```python
from build123d import *

# Parameters (mm, degrees)
SKETCH2_W           = 41
SKETCH2_H           = 35
BOSS_EXTRUDE1_DEPTH = 23.5
SKETCH3_W           = 30
SKETCH3_H           = 26
BOSS_EXTRUDE2_DEPTH = 5
SKETCH4_R           = 0.4
BOSS_EXTRUDE3_DEPTH = 2.5
CHAMFER1_SIZE       = 0.2


with BuildPart() as part:
    # Sketch2 → Boss-Extrude1 (new body)
    with BuildSketch(Plane(origin=(0, 0, 0), x_dir=(1, 0, 0), z_dir=(0, 1, 0))):
        Rectangle(SKETCH2_W, SKETCH2_H)
    extrude(amount=BOSS_EXTRUDE1_DEPTH)

    # Sketch3 → Boss-Extrude2 (add)
    with BuildSketch(Plane(origin=(0, 23.5, 0), x_dir=(1, 0, 0), z_dir=(0, 1, 0))):
        Rectangle(SKETCH3_W, SKETCH3_H)
    extrude(amount=BOSS_EXTRUDE2_DEPTH)

    # Sketch4 → Boss-Extrude3 (add)
    with BuildSketch(Plane.XZ):
        with Locations(Location((-10, 12.5, 0), (0, 0, 90))):
            Circle(SKETCH4_R)
        with Locations(Location((10, 12.5, 0), (0, 0, 90))):
            Circle(SKETCH4_R)
        with Locations(Location((-5, -12.5, 0), (0, 0, 90))):
            Circle(SKETCH4_R)
        with Locations(Location((5, -12.5, 0), (0, 0, 90))):
            Circle(SKETCH4_R)
    extrude(amount=BOSS_EXTRUDE3_DEPTH)

    # Chamfer1
    chamfer1_edges = [part.edges().sort_by_distance(p)[0] for p in [
        (20.5, 23.5, 0),
        (0, 23.5, -17.5),
        (15, 26, 13),
        (-15, 26, -13),
        (-15, 26, 13),
        (15, 28.5, 0),
        (0, 28.5, -13),
        (-15, 28.5, 0),
        (0, 28.5, 13),
        (-20.5, 23.5, 0),
        (0, 23.5, 17.5),
        (-20.5, 11.75, -17.5),
        (20.5, 11.75, -17.5),
        (20.5, 11.75, 17.5),
        (-20.5, 11.75, 17.5),
    ]]
    chamfer(chamfer1_edges, length=CHAMFER1_SIZE)


solid = part.part
```
For this review, take the finished solid that the model builds, in its own axes (mm). A direction names the side the tool comes from. Coordinates: 2 decimals unless noted, no trailing zeros. Write each loop counter-clockwise with the first axis right and the second up, starting at its lowest first coordinate (ties: lowest second). Pieces come first, ordered by that corner, then holes.
(1) Tool access review of faces 1 (the face through (0, 26, -13)), 2 (the face through (-15, 26, 0)), 3 (the face through (0, 26, 13)), 4 (the face through (0, 23.5, 15)): name each direction out of +Z, -Z, +X, -X, +Y, -Y from which nothing blocks a thin tool from reaching the whole face with its end or side.
(2) Add section C-C on z = -0.5. Give the boundary of the cut face in (x, y), then the cut area to 3 significant figures.
(3) Add section B-B on z = 15.5. Give the boundary of the cut face in (x, y), then the cut area to 3 significant figures.
(4) Wall thickness on probe 1 along Y at (x, z) = (-2, -4.5); probe 2 along X at (y, z) = (26.5, 7); probe 3 along Y at (x, z) = (17, -15): over which ranges is each line inside the solid? List them lowest first.
(5) For pin 1 Ø4 at (x, y) = (4, 26.5) entering from +Z; pin 2 Ø1.4 at (y, z) = (25, 3) entering from +X; pin 3 Ø8 at (x, z) = (0.5, 0.5) entering from -Y, all flat-tipped, find the tip position at first contact; note any pin that passes through.
(6) Add section A-A on x = 8. Give the boundary of the cut face in (y, z).
Answer sheet:
1. face 1: -Z, +X, -X, +Y
1. face 2: +Z, -Z, -X, +Y
1. face 3: +Z, +X, -X, +Y
1. face 4: +Y
2. outline: (-20.5, 0) - (20.5, 0) - (20.5, 23.3) - (20.3, 23.5) - (15, 23.5) - (15, 28.3) - (14.8, 28.5) - (-14.8, 28.5) - (-15, 28.3) - (-15, 23.5) - (-20.3, 23.5) - (-20.5, 23.3) - close
2. area: 1,110 mm2
3. outline: (-20.5, 0) - (20.5, 0) - (20.5, 23.3) - (20.3, 23.5) - (-20.3, 23.5) - (-20.5, 23.3) - close
3. area: 963 mm2
4. probe 1: y = 0 to 28.5
4. probe 2: x = -15 to 15
4. probe 3: y = 0 to 23.5
5. pin 1: stops at z = 13
5. pin 2: stops at x = 15
5. pin 3: stops at y = 0
6. outline: (0, -17.5) - (23.3, -17.5) - (23.5, -17.3) - (23.5, -13) - (28.3, -13) - (28.5, -12.8) - (28.5, 12.8) - (28.3, 13) - (23.5, 13) - (23.5, 17.3) - (23.3, 17.5) - (0, 17.5) - close
